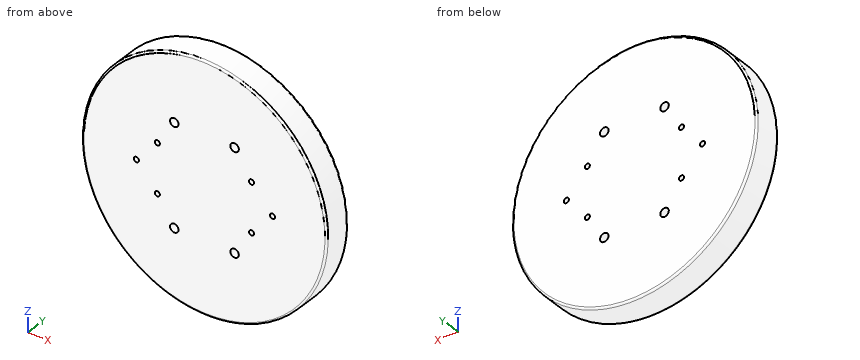
```python
from build123d import *

# Parameters (mm, degrees)
SKETCH1_R             = 65
BOSS_EXTRUDE1_DEPTH   = 15
FILLET1_R             = 1
F_6_32_TAPPED_HOLE1_D = 2.7051
F_8_CLEARANCE_HOLE1_D = 4.4958


with BuildPart() as part:
    # Sketch1 → Boss-Extrude1 (new body)
    with BuildSketch(Plane(origin=(0, 0, 0), x_dir=(1, 0, 0), z_dir=(0, 1, 0))):
        with Locations(Location((0, 0, 0), (0, 0, 270))):
            Circle(SKETCH1_R)
    extrude(amount=BOSS_EXTRUDE1_DEPTH)

    # Fillet1
    fillet1_edges = [part.edges().sort_by_distance(p)[0] for p in [
        (0, 0, -65),
        (0, 15, -65),
    ]]
    fillet(fillet1_edges, radius=FILLET1_R)

    # #6-32 Tapped Hole1 (through all)
    with Locations(Plane.XZ):
        with Locations((-36.145, 0), (36.145, 0), (-25, -13), (-25, 13), (25, 13), (25, -13)):
            Hole(F_6_32_TAPPED_HOLE1_D / 2)

    # #8 Clearance Hole1 (through all)
    with Locations(Plane(origin=(0, 0, 0), x_dir=(-1, 0, 0), z_dir=(0, -1, 0))):
        with Locations((16, -27), (-16, -27), (16, 27), (-16, 27)):
            Hole(F_8_CLEARANCE_HOLE1_D / 2)


solid = part.part
```
Read the model definition and answer for the solid it produces. Units are mm, in the model's axes. Coordinates: 2 decimals unless noted, no trailing zeros. Answer as a JSON object with one key per item and string values. Group by question number.
1. A cutting plane is placed at A-A (y = 10.25). Give the number of separate pieces and of enclosed holes in the cut face, plus the area to 3 significant figures.
2. Consider L1, parallel to X at y = 11.75, z = 27; L2, parallel to Z at x = 16, y = 4.75; L3, parallel to Z at x = 25, y = 4. Determine where each line is inside the solid, lowest interval first. Write a range as [from, to].
3. Each of these flat-tipped pins is pushed along its axis until it touches: P1, Ø2, axis at y = 10.5, z = 10, coming from the +X side; P2, Ø4, axis at y = 12, z = -7.5, coming from the -X side; P3, Ø5, axis at x = 16, z = 27, coming from the -Y side; P4, Ø2.5, axis at x = -25, z = -13, coming from the +Y side. Where does it stop, or does it pass through?
Worked out:
{
 "1": {"separate pieces": "1", "enclosed holes": "10", "area": "13,200 mm²"},
 "2": {"L1": "x = [-59.13, -18.25], [-13.75, 13.75], [18.25, 59.13]", "L2": "z = [-63, -29.25], [-24.75, 24.75], [29.25, 63]", "L3": "z = [-60, -14.35], [-11.65, 11.65], [14.35, 60]"},
 "3": {"P1": "stops at x = 64.37", "P2": "stops at x = -64.77", "P3": "stops at y = 0", "P4": "passes through"}
}
